```python
from build123d import *

# Parameters (mm, degrees)
PAD_DEPTH       = 19.3
POCKET_DEPTH    = 16.001
PAD001_DEPTH    = 2
SKETCH003_R     = 2.4
POCKET001_DEPTH = 3
CHAMFER_SIZE    = 0.3


with BuildPart() as part:
    # Sketch → Pad (new body)
    with BuildSketch(Plane.XY):
        Polygon((-9, 3), (-9, 9), (9, 9), (9, -9), (3, -9), align=None)
    extrude(amount=PAD_DEPTH)

    # Sketch001 (on DatumPlane) → Pocket (cut, through all)
    with BuildSketch(Plane.XY.offset(3.3)):
        Polygon((-9, 3), (3, 3), (3, -9), align=None)
    extrude(amount=POCKET_DEPTH, mode=Mode.SUBTRACT)

    # Sketch002 (on DatumPlane) → Pad001 (join)
    with BuildSketch(Plane.XY.offset(3.3)):
        with BuildLine():
            ThreePointArc((-3.8, 2.680869), (-3.3, 0.025), (-2.8, 2.680869))
            Line((-2.8, 2.680869), (-2.8, 3))
            Line((-3.8, 3), (-2.8, 3))
            Line((-3.8, 2.680869), (-3.8, 3))
        make_face()
        with BuildLine():
            ThreePointArc((2.680869, -2.8), (0.025, -3.3), (2.680869, -3.8))
            Line((3, -3.8), (2.680869, -3.8))
            Line((3, -2.8), (3, -3.8))
            Line((2.680869, -2.8), (3, -2.8))
        make_face()
    extrude(amount=PAD001_DEPTH)

    # Sketch003 → Pocket001 (cut)
    with BuildSketch(Plane.XY):
        with Locations((-0.3, -0.3)):
            Circle(SKETCH003_R)
    extrude(amount=POCKET001_DEPTH, mode=Mode.SUBTRACT)

    # Chamfer
    chamfer_edges = [part.edges().sort_by_distance(p)[0] for p in [
        (-3.3, 0.025, 5.3),
        (0.025, -3.3, 5.3),
    ]]
    chamfer(chamfer_edges, length=CHAMFER_SIZE)


solid = part.part
```
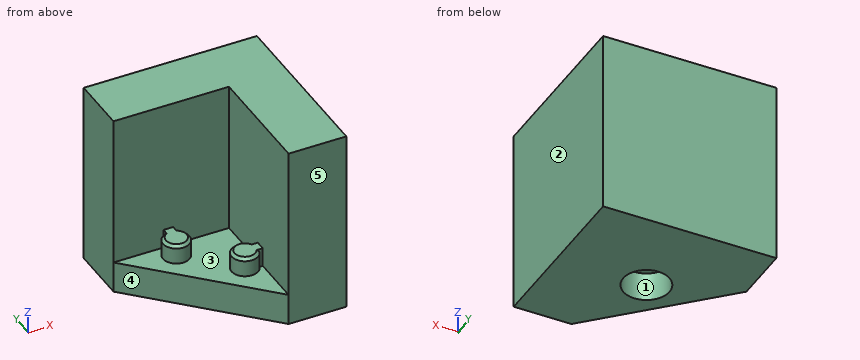
Geometry check sheet. Reference: the model listing, model coordinates, mm. Face numbers are marked on the shaded views. A direction names the side the tool comes from. Round coordinates to 2 decimals unless told otherwise and drop trailing zeros. Write each loop counter-clockwise with the first axis right and the second up, starting at its lowest first coordinate (ties: lowest second). Pieces come first, ordered by that corner, then holes. Notation, with made-up numbers: (-6, 40) -> (40, 40) arc R30 cw to (40, 64) -> close; hole circle Ø6 at (-17.75, -3.75). An arc over 180 degrees is marked (long way). Put each result on its own line as item: value.
1) Cross-section at B-B, the plane z = 2. Enter the section's corners in (x, y), plus the area to 3 significant figures.
Recorded:
outline: (-9, 3) -> (3, -9) -> (9, -9) -> (9, 9) -> (-9, 9) -> close; hole circle Ø4.8 at (-0.3, -0.3)
area: 234 mm2
2) Access from +Z, -Z, +X, -X, +Y, -Y to the whole of each face (thin tool, end or side, straight path). Record for the marked faces 1 and 2.
Recorded:
face 1: -Z
face 2: +Z, -Z, +X, +Y, -Y
3) Release check for a two-part mould opening along X. For the marked faces 3, 4 and 5 record: pulls with the +X half, pulls with the -X half, needs draft (parallel to the pull), parting line crosses it, or undercut.
Recorded:
face 3: undercut
face 4: pulls with the -X half
face 5: needs draft
4) Cross-section at A-A, the plane y = -3.3. Enter the section's corners in (x, z) (3 decimals), plus the area to 3 significant figures.
Recorded:
outline: (-2.7, 0) -> (9, 0) -> (9, 19.3) -> (3, 19.3) -> (3, 5.3) -> (0.325, 5.3) -> (0.025, 5) -> (0.025, 3.3) -> (-2.7, 3.3) -> close
area: 141 mm2
5) Depth check by flat-ended pin: P1, Ø9.5, axis at x = -5, z = 11, coming from the -Y side; P2, Ø6, axis at x = -2.5, y = -6, coming from the +Z side; P3, Ø6, axis at y = -4, z = 10, coming from the -X side. Enter the tip coordinate at first touch or a pass-through.
Recorded:
P1: stops at y = 3
P2: stops at z = 3.3
P3: stops at x = 3
6) Thickness scan on probe 1 along X at (y, z) = (-5.5, 18.25); probe 2 along Y at (x, z) = (-0.3, 1). Record the ranges inside material, lowest first. Write a range as from..to.
Recorded:
probe 1: x = 3..9
probe 2: y = -5.7..-2.7, 2.1..9
7) Cross-section at D-D, the plane z = 6. Enter the section's corners in (x, y), plus the area to 3 significant figures.
Recorded:
outline: (-9, 3) -> (3, 3) -> (3, -9) -> (9, -9) -> (9, 9) -> (-9, 9) -> close
area: 180 mm2
